Autodesk Inventor part; units mm, degrees
ref_plane "YZ Plane" through (0, 0, 0) normal (1, 0, 0) x (0, 1, 0)
ref_plane "XZ Plane" through (0, 0, 0) normal (0, 1, 0) x (-1, 0, 0)
ref_plane "XY Plane" through (0, 0, 0) normal (0, 0, 1) x (1, 0, 0)
sketch "Sketch1" plane through (0, 0, 0) normal (0, 1, 0) x (-1, 0, 0)
  line L0 (9.5, 29) -> (-9.5, 29)
  line L1 (-9.5, -26.5) -> (-7.9373, -26.5)
  line L2 (10, 0) -> (10, 15)
  line L3 (10, 15) -> (11.5, 15)
  line L4 (12, 15.5) -> (12, 18.5)
  line L5 (11.5, 19) -> (10, 19)
  line L6 (10, 0) -> (10, -15)
  line L7 (10, -15) -> (11.5, -15)
  line L8 (12, -15.5) -> (12, -18.5)
  line L9 (11.5, -19) -> (10, -19)
  line L10 (-10, 0) -> (-10, 15)
  line L11 (-10, 15) -> (-11.5, 15)
  line L12 (-12, 15.5) -> (-12, 18.5)
  line L13 (-11.5, 19) -> (-10, 19)
  line L14 (-10, 0) -> (-10, -15)
  line L15 (-10, -15) -> (-11.5, -15)
  line L16 (-12, -15.5) -> (-12, -18.5)
  line L17 (-11.5, -19) -> (-10, -19)
  line L18 (10, 19) -> (10, 28.5)
  line L19 (10, -19.5) -> (10, -19)
  line L20 (10, -15) -> (10, 15)
  line L21 (-10, -19) -> (-10, -19.5)
  line L22 (-10, 28.5) -> (-10, 19)
  line L23 (-10, 15) -> (-10, -15)
  arc A0 (11.5, 15) -> (12, 15.5) centre (11.5, 15.5) ccw
  arc A1 (12, 18.5) -> (11.5, 19) centre (11.5, 18.5) ccw
  arc A2 (-11.5, 19) -> (-12, 18.5) centre (-11.5, 18.5) ccw
  arc A3 (-12, 15.5) -> (-11.5, 15) centre (-11.5, 15.5) ccw
  arc A4 (12, -15.5) -> (11.5, -15) centre (11.5, -15.5) ccw
  arc A5 (11.5, -19) -> (12, -18.5) centre (11.5, -18.5) ccw
  arc A6 (-11.5, -15) -> (-12, -15.5) centre (-11.5, -15.5) ccw
  arc A7 (-12, -18.5) -> (-11.5, -19) centre (-11.5, -18.5) ccw
  line L24 (0, -26.5) -> (0, -35.5) construction
  arc A8 (7.9373, -26.5) -> (-7.9373, -26.5) centre (0, -35.5) ccw
  arc A9 (10, 28.5) -> (9.5, 29) centre (9.5, 28.5) ccw
  arc A10 (-9.5, 29) -> (-10, 28.5) centre (-9.5, 28.5) ccw
  line L25 (7.9373, -26.5) -> (9.5, -26.5)
  line L26 (-7.9373, -26.5) -> (7.9373, -26.5) construction
  line L27 (0, -26.5) -> (0, -26.5) construction
  line L28 (10, -19.5) -> (10, -26)
  line L29 (9.5, -26.5) -> (9.5, -26.5)
  line L30 (-10, -19.5) -> (-10, -26)
  line L31 (-9.5, -26.5) -> (-9.5, -26.5)
  arc A11 (9.5, -26.5) -> (10, -26) centre (9.5, -26) ccw
  arc A12 (-10, -26) -> (-9.5, -26.5) centre (-9.5, -26) ccw
  line L32 (0, 29) -> (0, 29) construction
  point P0 (0, 0)
  point P1 (12, 15)
  point P2 (12, 19)
  point P3 (12, -15)
  point P4 (12, -19)
  point P5 (-12, 15)
  point P6 (-12, 19)
  point P7 (-12, -15)
  point P8 (-12, -19)
  point P9 (-10, -26.5)
  dimension "d2" = 15
  dimension "d3" = 2
  dimension "d4" = 4
  dimension "d5" = 15
  dimension "d6" = 4
  dimension "d7" = 15
  dimension "d8" = 2
  dimension "d9" = 4
  dimension "d10" = 15
  dimension "d11" = 4
  dimension "d12" = 0.5
  dimension "d13" = 9
  dimension "d14" = 12
  dimension "d15" = 0.5
  dimension "d26" = 0
  dimension "d27" = 0.5
  dimension "d28" = 0
extrude "Extrusion1" add sketch "Sketch1" along normal blind 2
sketch "Sketch2" plane through (0, 2, 0) normal (0, 1, 0) x (1, 0, 0)
  line L0 (-4, 16.2872) -> (4, 16.2872) construction
  line L1 (-4, 15.2872) -> (4, 15.2872)
  line L2 (4, 17.2872) -> (-4, 17.2872)
  arc A0 (-4, 17.2872) -> (-4, 15.2872) centre (-4, 16.2872) ccw
  arc A1 (4, 15.2872) -> (4, 17.2872) centre (4, 16.2872) ccw
  line L3 (0, 20.2872) -> (0, 12.2872) construction
  line L4 (-1, 20.2872) -> (-1, 12.2872)
  line L5 (1, 12.2872) -> (1, 20.2872)
  arc A2 (1, 20.2872) -> (-1, 20.2872) centre (0, 20.2872) ccw
  arc A3 (-1, 12.2872) -> (1, 12.2872) centre (0, 12.2872) ccw
  line L6 (0, 16.2872) -> (0, 21.2872) construction
  point P0 (0, 0)
  point P1 (-1, 15.2872)
  point P2 (1, 15.2872)
  point P3 (1, 17.2872)
  point P4 (-1, 17.2872)
  point P5 (0, 21.2872)
  dimension "d18" = 4
  dimension "d19" = 2
  dimension "d20" = 4
  dimension "d21" = 2
  dimension "d29" = 5
extrude "Extrusion2" cut sketch "Sketch2" against normal blind 2
properties part number "Laser-Slot-Top" material "Acrylic, Clear"
Source: CAD feature listing. Evaluate the final solid. Frame: model axes, mm. A direction names the side the tool comes from. Round coordinates to 2 decimals unless told otherwise and drop trailing zeros. Write each loop counter-clockwise with the first axis right and the second up, starting at its lowest first coordinate (ties: lowest second). Pieces come first, ordered by that corner, then holes. Notation, with made-up numbers: M -11.5,47.25 L 2.5,47.25 A30 ccw 2.5,75.25 Z; hole C 66.5,86.25 d2. An arc over 180 degrees is marked long. Use CSV: the item, a comma, the result in double quotes. Start each with the question number.
Q1. Access query for faces 4 (the face through (11, 1, -15)), 5 (the face through (-0.022, 1.014, -11.287)), 6 (the face through (10, 1, 24)), 7 (the face through (11, 1, -19)). Directions: +Z, -Z, +X, -X, +Y, -Y. A direction counts if a zero-diameter tool reaches every point of the face in a straight line with its end or side. Return the directions, or none.
Q2. Cut plane D-D on x = 6.5. Output: boundary loops of the cut face in (y, z), plus the area to 3 significant figures.
Q3. Cut plane C-C on z = -2.5. Output: boundary loops of the cut face in (x, y).
Q4. Pull-direction query (X, two-part tool) for faces 1 (the face through (-11, 1, -19)), 2 (the face through (1, 1, -19)), 3 (the face through (12, 1, -17)); classes: +X half, -X half, draft (parallel to the pull), parting line (faces both ways), or undercut.
Q5. Cut plane A-A on z = -13. Output: boundary loops of the cut face in (x, y).
Q6. Cut plane B-B on x = 0. Output: boundary loops of the cut face in (y, z), plus the area to 3 significant figures.
Q7. First-contact query: P1, Ø1, axis at y = 1.5, z = -1.5, coming from the -X side; P2, Ø1, axis at y = 1.5, z = -13.5, coming from the +X side. Flat tips, straight axial feed; report the tip coordinate or a pass-through.
Q8. Line query: line 1 (Z direction, x = -10.5, y = 1.6); line 2 (X direction, y = 0.6, z = -13); line 3 (Z direction, x = 1.25, y = 0.3). Output: solid intervals per line, ascending. Write a range as from..to.
Results found:
1,face 4,"+X, +Y, -Y"
1,face 5,"+Y, -Y"
1,face 6,"+Z, +X, +Y, -Y"
1,face 7,"-Z, +X, +Y, -Y"
2,outline,"M 0,-25.41 L 2,-25.41 L 2,29 L 0,29 Z"
2,area,"109 mm^2"
3,outline,"M -10,0 L 10,0 L 10,2 L -10,2 Z"
4,face 1,"draft"
4,face 2,"undercut"
4,face 3,"+X half"
5,outline,"M -10,0 L -1,0 L -1,2 L -10,2 Z; M 1,0 L 10,0 L 10,2 L 1,2 Z"
6,outline,"M 0,-23.5 L 2,-23.5 L 2,-21.29 L 0,-21.29 Z; M 0,-11.29 L 2,-11.29 L 2,29 L 0,29 Z"
6,area,"85.0 mm^2"
7,P1,"x = -10"
7,P2,"x = 10"
8,line 1,"-19..-15, 15..19"
8,line 2,"-10..-1, 1..10"
8,line 3,"-23.57..-17.29, -15.29..29"
